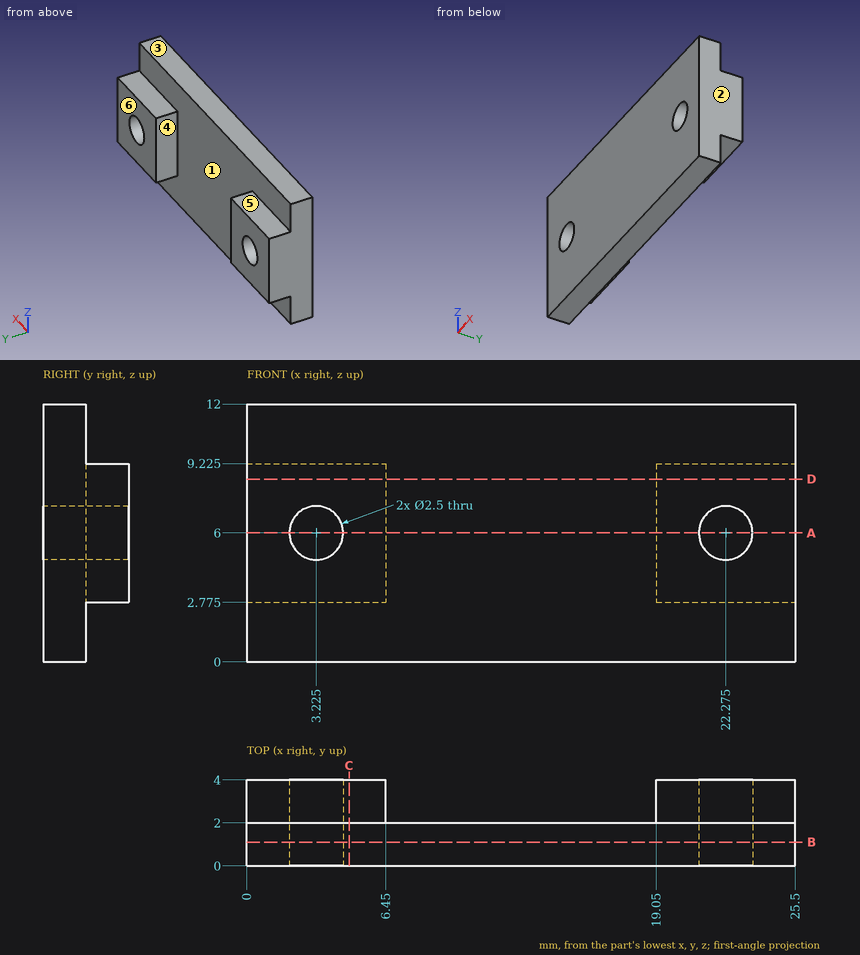
Could you check a few things on this drawing? It's one solid part, dimensions in mm from its lowest x, y, z. A direction names the side the tool comes from. Coordinates: 2 decimals unless noted, no trailing zeros. Write each loop counter-clockwise with the first axis right and the second up, starting at its lowest first coordinate (ties: lowest second). Pieces come first, ordered by that corner, then holes.
Q1. Please list where these lines run through material, in increasing order: L1, parallel to X at y = 1.2, z = 6 (3 decimals); L2, parallel to X at y = 2.95, z = 6 (3 decimals); L3, parallel to X at y = 3.4, z = 5 (3 decimals).
Results found:
L1: x = 0 to 1.975, 4.475 to 21.025, 23.525 to 25.5
L2: x = 0 to 1.975, 4.475 to 6.45, 19.05 to 21.025, 23.525 to 25.5
L3: x = 0 to 2.475, 3.975 to 6.45, 19.05 to 21.525, 23.025 to 25.5
Q2. Imagine slicing it at B-B, the plane y = 1.1. List the corners of the cut face in (x, z) for me (3 decimals), plus the area to 3 significant figures.
Results found:
outline: (0, 0) - (25.5, 0) - (25.5, 12) - (0, 12) - close; hole circle Ø2.5 at (3.225, 6); hole circle Ø2.5 at (22.275, 6)
area: 296 mm2
Q3. If we mould it in two halves opening along X, with no side actions, what happens to the marked faces 1, 2, 3 and 4? For each: +X half, -X half, draft (parallel to the pull), parting line (faces both ways), or undercut.
Results found:
face 1: undercut
face 2: +X half
face 3: draft
face 4: undercut
Q4. Which directions (+Z, -Z, +X, -X, +Y, -Y) give clear straight access to the entire face, cutting with the end or side of a thin tool? Please do the marked faces 5 and 6.
Results found:
face 5: +Z, +X, -X, +Y
face 6: +Z, -Z, +X, -X, +Y
Q5. Imagine slicing it at A-A, the plane z = 6. List the corners of the cut face in (x, y) for me (3 decimals).
Results found:
outline: (0, 0) - (1.975, 0) - (1.975, 4) - (0, 4) - close; (4.475, 0) - (21.025, 0) - (21.025, 4) - (19.05, 4) - (19.05, 2) - (6.45, 2) - (6.45, 4) - (4.475, 4) - close; (23.525, 0) - (25.5, 0) - (25.5, 4) - (23.525, 4) - close
Q6. Imagine slicing it at D-D, the plane z = 8.5. List the corners of the cut face in (x, y) for me, plus the area to 3 significant figures.
Results found:
outline: (0, 0) - (25.5, 0) - (25.5, 4) - (19.05, 4) - (19.05, 2) - (6.45, 2) - (6.45, 4) - (0, 4) - close
area: 76.8 mm2
Q7. For P1, Ø2, axis at x = 21.5, y = 3.5, coming from the -Z side (3 decimals); P2, Ø3, axis at x = 3.225, z = 6, coming from the -Y side; P3, Ø6, axis at x = 13.5, z = 8, coming from the +Y side; P4, Ø0.6, axis at x = 23, y = 3.5, coming from the +Z side (3 decimals), each with a flat end and sliding along its axis, tell me the tip position at first contact or that it passes through.
Results found:
P1: stops at z = 2.775
P2: stops at y = 0
P3: stops at y = 2
P4: stops at z = 9.225
Q8. Imagine slicing it at C-C, the plane x = 4.75. List the corners of the cut face in (y, z) for me (3 decimals), plus the area to 3 significant figures.
Results found:
outline: (0, 0) - (2, 0) - (2, 2.775) - (4, 2.775) - (4, 9.225) - (2, 9.225) - (2, 12) - (0, 12) - close
area: 36.9 mm2
